from build123d import *

# Parameters (mm, degrees)
EXTRUDE_1_DEPTH = 6
FILLET_1_R      = 0.5
FILLET_2_R      = 2
FILLET_3_R      = 1


with BuildPart() as part:
    # 草圖1 → 填料-伸長1 (new body)
    with BuildSketch(Plane.XY):
        Polygon((-48.713400366, 0), (-41.70660185, 0), (-41.70660185, -4.56), (-46.70660185, -4.56), (-46.70660185, -2.007214056), (-48.713400366, -2.007214056), align=None)
    extrude(amount=EXTRUDE_1_DEPTH)

    # 圓角1
    fillet_1_edges = [part.edges().sort_by_distance(p)[0] for p in [
        (-41.70660185, 0, 3),
    ]]
    fillet(fillet_1_edges, radius=FILLET_1_R)

    # 圓角2
    fillet_2_edges = [part.edges().sort_by_distance(p)[0] for p in [
        (-48.713400366, 0, 3),
    ]]
    fillet(fillet_2_edges, radius=FILLET_2_R)

    # 圓角3
    fillet_3_edges = [part.edges().sort_by_distance(p)[0] for p in [
        (-46.70660185, -2.007214056, 3),
    ]]
    fillet(fillet_3_edges, radius=FILLET_3_R)


solid = part.part
Input: part model. Units: mm. Frame: model coordinates. A direction names the side the tool comes from. Give positions to 0.01 mm unless a question says otherwise; leave off trailing zeros. Write each loop counter-clockwise with the first axis right and the second up, starting at its lowest first coordinate (ties: lowest second). Pieces come first, ordered by that corner, then holes.
Q1. Section C-C, the plane x = -48. Output: boundary loops of the cut face in (y, z).
Q2. Section B-B, the plane y = -3.55. Output: boundary loops of the cut face in (x, z).
Q3. Material intervals for probe 1 along X at (y, z) = (-4.1, 5); probe 2 along X at (y, z) = (-1.9, 3.75); probe 3 along Y at (x, z) = (-48.5, 2.05), sorted ascending.
Q4. First-contact query: P1, Ø1, axis at x = -45.5, y = -3.5, coming from the -Z side; P2, Ø1.7, axis at y = -4, z = 2, coming from the -X side. Flat tips, straight axial feed; report the tip coordinate or a pass-through.
Q5. Set-up query: faces 1 (the face through (-44, -4.56, 3)), 2 (the face through (-46.707, -4, 3)). Return all of +Z, -Z, +X, -X, +Y, -Y with unobstructed straight access to the full face (end or side cutting, diameter ignored); none if empty.
Filled in:
1. outline: (-2.01, 0) - (-0.47, 0) - (-0.47, 6) - (-2.01, 6) - close
2. outline: (-46.71, 0) - (-41.71, 0) - (-41.71, 6) - (-46.71, 6) - close
3. probe 1: x = -46.71 to -41.71
3. probe 2: x = -48.71 to -41.71
3. probe 3: y = -2.01 to -1.1
4. P1: stops at z = 0
4. P2: stops at x = -46.71
5. face 1: +Z, -Z, +X, -X, -Y
5. face 2: +Z, -Z, -X, -Y
